Can you work these out from the model? Positions are in its coordinate system, mm. Give positions to 0.01 mm unless a question says otherwise; leave off trailing zeros. Order: outer loops, then holes, each group sorted by start corner. A loop starts at its lowest first (then second) coordinate and runs counter-clockwise, first axis right, second up. Notation, with made-up numbers: M 0.25,14.25 L 34.25,14.25 A22 cw 34.25,38.25 Z; hole C -24.75,-33 d11. An arc over 180 degrees is marked long. Use one line per item in the form item = value. Start each with the question number.
1. Will these pins go through, and if not, where does the flat tip stop? P1, Ø6, axis at x = 158.75, z = -57.15, coming from the +Y side; P2, Ø12, axis at x = -5, z = 147.5, coming from the -Y side; P3, Ø3, axis at x = -100.5, y = 3.5, coming from the +Z side.
2. I want a section at B-B, the plane y = 3.25. Count the separate pieces of the cut face and the enclosed holes in it, and give its area (3 significant figures).
3. I need wall thicknesses on L1, parallel to X at y = 3.5, z = -158.75; L2, parallel to Z at x = 158.75, y = 4; L3, parallel to X at y = 1.5, z = 146.05. Which ranges of each line are inside material? Lowest first, please.
4. We'd pull the mould along X, two halves only. Please class faces 1 (the face through (-29.439, 3.219, 196.904)), 2 (the face through (41.485, 3.131, 131.735)), 3 (the face through (-2, 0, -147)): +X half, -X half, draft (parallel to the pull), parting line (faces both ways), or undercut.
5. I want a section at A-A, the plane z = 0. List the corners of the cut face in (x, y) for me.
```python
from build123d import *

# Parameters (mm, degrees)
SKETCH1_R               = 138.1125
SKETCH1_R_2             = 14.2875
BOSS_EXTRUDE1_DEPTH     = 6.35
FILLET1_R               = 25.4
FILLET2_R               = 31.75
F_3_8_CLEARANCE_HOLE1_D = 10.0838
F_1_4_CLEARANCE_HOLE1_D = 6.7564
FILLET3_R               = 6.35
SKETCH2_R               = 2.38125


with BuildPart() as part:
    # Sketch1 → Boss-Extrude1 (new body)
    with BuildSketch(Plane(origin=(0, 0, 0), x_dir=(1, 0, 0), z_dir=(0, 1, 0))):
        Polygon((38.1, -152.4), (165.1, -152.4), (165.1, 165.1), (-165.1, 165.1), (-165.1, -152.4), (-38.1, -152.4), (-38.1, -203.2), (38.1, -203.2), align=None)
        with Locations(Location((0, 0, 0), (0, 0, 270))):
            Circle(SKETCH1_R, mode=Mode.SUBTRACT)
        with Locations(Location((0, -174.625, 0), (0, 0, 270))):
            Circle(SKETCH1_R_2, mode=Mode.SUBTRACT)
    extrude(amount=BOSS_EXTRUDE1_DEPTH)

    # Fillet1
    fillet1_edges = [part.edges().sort_by_distance(p)[0] for p in [
        (38.1, 3.175, 203.2),
        (-38.1, 3.175, 203.2),
    ]]
    fillet(fillet1_edges, radius=FILLET1_R)

    # Fillet2
    fillet2_edges = [part.edges().sort_by_distance(p)[0] for p in [
        (38.1, 3.175, 152.4),
        (-38.1, 3.175, 152.4),
    ]]
    fillet(fillet2_edges, radius=FILLET2_R)

    # 3_8 Clearance Hole1 (through all)
    with Locations(Plane(origin=(0, 0, 0), x_dir=(-1, 0, 0), z_dir=(0, -1, 0))):
        with Locations((34.925, -158.75), (-34.925, -158.75)):
            Hole(F_3_8_CLEARANCE_HOLE1_D / 2)

    # 1_4 Clearance Hole1 (through all)
    with Locations(Plane(origin=(0, 6.35, 0), x_dir=(1, 0, 0), z_dir=(0, 1, 0))):
        with Locations((158.75, 158.75), (-158.75, 158.75), (158.75, 57.15), (-158.75, 57.15), (158.75, -44.45), (-158.75, -44.45), (158.75, -146.05), (-158.75, -146.05), (-57.15, 158.75), (57.15, 158.75)):
            Hole(F_1_4_CLEARANCE_HOLE1_D / 2)

    # Fillet3
    fillet3_edges = [part.edges().sort_by_distance(p)[0] for p in [
        (165.1, 3.175, 152.4),
        (-165.1, 3.175, 152.4),
        (-165.1, 3.175, -165.1),
        (165.1, 3.175, -165.1),
    ]]
    fillet(fillet3_edges, radius=FILLET3_R)

    # Sketch2 → Cut-Revolve1 (revolve, cut)
    with BuildSketch(Plane(origin=(0, 0, 0), x_dir=(0, 0, -1), z_dir=(1, 0, 0)), mode=Mode.PRIVATE) as cut_revolve1_sk:
        with Locations((-141.2875, 7.14375)):
            Circle(SKETCH2_R)
        with Locations((-141.2875, -0.79375)):
            Circle(SKETCH2_R)
    revolve(cut_revolve1_sk.sketch.rotate(Axis((0, 0, 0), (0, 1, 0)), 180), axis=Axis((0, 0, 0), (0, 1, 0)), mode=Mode.SUBTRACT)


solid = part.part
```
Check result:
q1.P1 = through
q1.P2 = 0
q1.P3 = 152.4
q2.separate_pieces = 1
q2.enclosed_holes = 14
q2.area = 47,700 mm2
q3.L1 = -165.1 to -162.13, -155.37 to -60.53, -53.77 to 53.77, 60.53 to 155.37, 162.13 to 165.1
q3.L2 = -165.1 to -162.13, -155.37 to -60.53, -53.77 to 41.07, 47.83 to 142.67, 149.43 to 152.4
q3.L3 = -165.1 to -162.13, -155.37 to 155.37, 162.13 to 165.1
q4.face_1 = -X half
q4.face_2 = undercut
q4.face_3 = draft
q5.outline = M -165.1,0 L -143.53,0 A2.38 cw -139.04,0 L -138.11,0 L -138.11,6.35 L -139.04,6.35 A2.38 cw -143.53,6.35 L -165.1,6.35 Z; M 138.11,0 L 139.04,0 A2.38 cw 143.53,0 L 165.1,0 L 165.1,6.35 L 143.53,6.35 A2.38 cw 139.04,6.35 L 138.11,6.35 Z
